```python
from build123d import *

# Parameters (mm, degrees)
SKETCH_1_R      = 1.229324964
SKETCH_1_R_2    = 1.149420027
EXTRUDE_1_DEPTH = 2
SKETCH_2_R      = 7.221294113
EXTRUDE_2_DEPTH = 4
SKETCH_3_W      = 2.645095026
SKETCH_3_H      = 3.141050342
SKETCH_3_W_2    = 1.884630206
SKETCH_3_H_2    = 3.041859279
SKETCH_3_W_3    = 1.96408086
SKETCH_3_H_3    = 3.372496157
SKETCH_3_W_4    = 2.57896765
SKETCH_3_H_4    = 3.008795591
EXTRUDE_3_DEPTH = 2.5


with BuildPart() as part:
    # 草图1 → 凸台-拉伸1 (new body)
    with BuildSketch(Plane(origin=(0, 0, 0), x_dir=(1, 0, 0), z_dir=(0, 1, 0))):
        Polygon((-27.440284042, -0.784220791), (20.007371412, -0.784220791), (20.007371412, -16.804782103), (14.704398156, -18.535226008), (5.996357861, -19.819103743), (1.753979255, -20.209849141), (-1.651087783, -20.209849141), (-12.703600465, -19.428358346), (-21.802386158, -19.428358346), (-22.695518496, -18.535226008), (-27.440284042, -18.535226008), align=None)
        with Locations(Location((-24.537603943, -16.023291307, 0), (0, 0, 270))):
            Circle(SKETCH_1_R, mode=Mode.SUBTRACT)
        with Locations(Location((3.093677762, -3.072872407, 0), (0, 0, 270))):
            Circle(SKETCH_1_R_2, mode=Mode.SUBTRACT)
    extrude(amount=EXTRUDE_1_DEPTH)

    # 草图2 → 凸台-拉伸2 (add)
    with BuildSketch(Plane(origin=(0, 2, 0), x_dir=(1, 0, 0), z_dir=(0, 1, 0))):
        with Locations(Location((10.864630012, -9.521656176, 0), (0, 0, 270))):
            Circle(SKETCH_2_R)
    extrude(amount=EXTRUDE_2_DEPTH)

    # 草图3 → 凸台-拉伸3 (add)
    with BuildSketch(Plane(origin=(0, 0, 0), x_dir=(-1, 0, 0), z_dir=(0, -1, 0))):
        with Locations((24.315133823, -7.322920936)):
            Rectangle(SKETCH_3_W, SKETCH_3_H)
        with Locations((9.552197214, -7.736217034)):
            Rectangle(SKETCH_3_W_2, SKETCH_3_H_2)
        with Locations((0.98204043, -7.901535473)):
            Rectangle(SKETCH_3_W_3, SKETCH_3_H_3)
        with Locations((-11.029948451, -8.083385756)):
            Rectangle(SKETCH_3_W_4, SKETCH_3_H_4)
    extrude(amount=EXTRUDE_3_DEPTH)


solid = part.part
```
The model under review builds one solid part; all positions refer to its coordinate system, in mm. A direction names the side the tool comes from. Round coordinates to 2 decimals unless told otherwise and drop trailing zeros. Loops run counter-clockwise (first coordinate to the right, second up) from the corner with the lowest first, then second, coordinate; pieces in that order, holes last.
Item 1: Take a section at D-D (z = 5.25). Write out the cut boundary in (x, y), then the cut area to 3 significant figures.
Determined:
outline: (-27.44, 0) - (20.01, 0) - (20.01, 2) - (16.69, 2) - (16.69, 6) - (5.04, 6) - (5.04, 2) - (-27.44, 2) - close
area: 141 mm2
Item 2: Mouldability with a two-part tool opening along Z and no side actions: class faces 5 (the face through (2.653, 0.986, 4.135)), 6 (the face through (-4, 1, 0.784)), 7 (the face through (-22.993, -1, 7)) as released by +Z, released by -Z, zero draft, split by the parting line, or undercut.
Determined:
face 5: undercut
face 6: released by -Z
face 7: zero draft
Item 3: Take a section at C-C (x = 8). Write out the cut boundary in (y, z).
Determined:
outline: (0, 0.78) - (2, 0.78) - (2, 2.89) - (6, 2.89) - (6, 16.15) - (2, 16.15) - (2, 19.52) - (0, 19.52) - close
Item 4: Clearance check with flat-ended pins moving along their axes: pin 1 Ø1.2 at (x, y) = (11.5, -1.5) entering from +Z; pin 2 Ø3 at (x, y) = (-24, -1) entering from +Z; pin 3 Ø1.2 at (y, z) = (-2, 8.5) entering from -X; pin 4 Ø1 at (x, y) = (-4, 4) entering from +Z. State where each tip first meets the part, or that it passes through.
Determined:
pin 1: stops at z = 9.59
pin 2: stops at z = 18.54
pin 3: stops at x = -25.64
pin 4: passes through
Item 5: Take a section at A-A (y = -0.75). Write out the cut boundary in (x, z), then the cut area to 3 significant figures.
Determined:
outline: (-25.64, 5.75) - (-22.99, 5.75) - (-22.99, 8.89) - (-25.64, 8.89) - close; (-10.49, 6.22) - (-8.61, 6.22) - (-8.61, 9.26) - (-10.49, 9.26) - close; (-1.96, 6.22) - (0, 6.22) - (0, 9.59) - (-1.96, 9.59) - close; (9.74, 6.58) - (12.32, 6.58) - (12.32, 9.59) - (9.74, 9.59) - close
area: 28.4 mm2
Item 6: For faces 1 (the face through (-10, -1, 9.257)), 2 (the face through (-1, -1, 6.215)), 3 (the face through (11, -1, 9.588)), 4 (the face through (-24, -1, 5.752)), list the 3-axis set-ups (+Z, -Z, +X, -X, +Y, -Y) from which the entire face can be reached by the end or side of a thin tool; tool diameter is ignored.
Determined:
face 1: +Z, -X, -Y
face 2: -Z, +X, -Y
face 3: +Z, +X, -X, -Y
face 4: -Z, +X, -X, -Y
Item 7: For line 1 (Y direction, x = -10, z = 4.5); line 2 (Z direction, x = -9.5, y = -1); line 3 (Z direction, x = -21, y = 1.5), list the stretches that pass through material, from the lowest coordinate up.
Determined:
line 1: y = 0 to 2
line 2: z = 6.22 to 9.26
line 3: z = 0.78 to 19.43
Item 8: Take a section at B-B (z = 3). Write out the cut boundary in (x, y), then the cut area to 3 significant figures.
Determined:
outline: (-27.44, 0) - (1.95, 0) - (1.95, 2) - (-27.44, 2) - close; (4.24, 0) - (20.01, 0) - (20.01, 2) - (13.97, 2) - (13.97, 6) - (7.76, 6) - (7.76, 2) - (4.24, 2) - close
area: 115 mm2
